Geometry: see drawing. Coordinates: mm, zero at the bounding-box minimum. A direction names the side the tool comes from. Give positions to 0.01 mm unless a question says otherwise; leave off trailing zeros. Loops run counter-clockwise (first coordinate to the right, second up) from the corner with the lowest first, then second, coordinate; pieces in that order, holes last. Notation, with made-up numbers: M 33.25,-28 L 57.25,-28 A26 cw 57.25,-10 Z; hole C 10,83 d3. An arc over 180 degrees is marked long. Return JSON: item names as keys, results as strings. Group by question number.
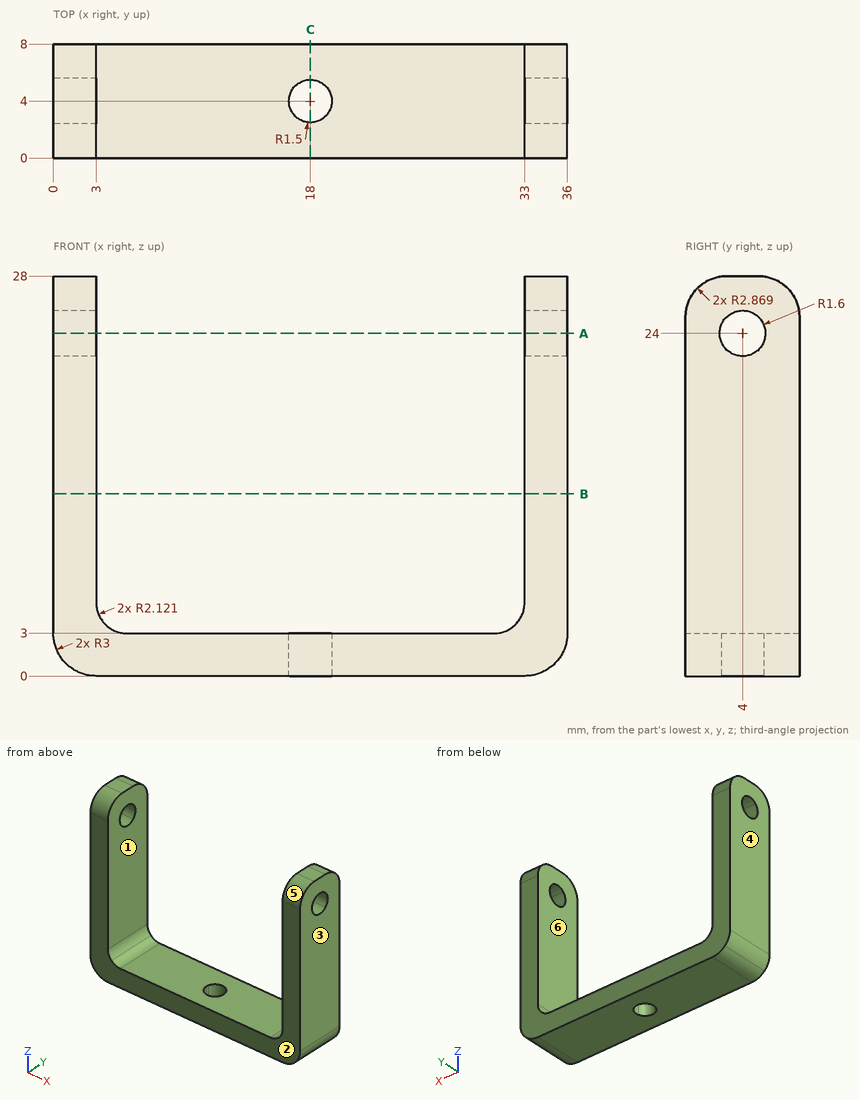
Item 1: Reachability of the marked faces 1 and 2 from +Z, -Z, +X, -X, +Y, -Y: full face, straight path, thin tool, end or side. Return the list, or none.
Item 2: Section B-B, the plane z = 12.75. Return loops of the section in (x, y), then the cut area to 3 significant figures.
Item 3: First-contact query: pin 1 Ø4 at (x, y) = (17, 4) entering from +Z. Flat tip, straight axial feed; report the tip coordinate or a pass-through.
Item 4: Section C-C, the plane x = 18. Return loops of the section in (y, z), then the cut area to 3 significant figures.
Item 5: Material intervals for line 1 (X direction, y = 4.75, z = 6.5); line 2 (Z direction, x = 26.5, y = 5.75); line 3 (X direction, y = 1, z = 2.25) (1 decimal), sorted ascending. Write a range as from..to.
Item 6: Section A-A, the plane z = 24. Return loops of the section in (x, y).
Item 7: Pull-direction query (X, two-part tool) for the marked faces 3, 4, 5 and 6; classes: pulls with the +X half, pulls with the -X half, needs draft (parallel to the pull), parting line crosses it, or undercut.
Answer below:
{
 "1": {"face 1": "+Z, +Y, -Y", "face 2": "+Z, -Z, +X, -X, -Y"},
 "2": {"outline": "M 0,0 L 3,0 L 3,8 L 0,8 Z; M 33,0 L 36,0 L 36,8 L 33,8 Z", "area": "48.0 mm^2"},
 "3": {"pin 1": "z = 3"},
 "4": {"outline": "M 0,0 L 2.5,0 L 2.5,3 L 0,3 Z; M 5.5,0 L 8,0 L 8,3 L 5.5,3 Z", "area": "15.0 mm^2"},
 "5": {"line 1": "0..3, 33..36", "line 2": "0..3", "line 3": "0.1..35.9"},
 "6": {"outline": "M 0,0 L 3,0 L 3,2.4 L 0,2.4 Z; M 0,5.6 L 3,5.6 L 3,8 L 0,8 Z; M 33,0 L 36,0 L 36,2.4 L 33,2.4 Z; M 33,5.6 L 36,5.6 L 36,8 L 33,8 Z"},
 "7": {"face 3": "pulls with the +X half", "face 4": "pulls with the -X half", "face 5": "needs draft", "face 6": "undercut"}
}
